Read the model definition and answer for the solid it produces. Units are mm, in the model's axes. A direction names the side the tool comes from. Round coordinates to 2 decimals unless told otherwise and drop trailing zeros. Write each loop counter-clockwise with the first axis right and the second up, starting at its lowest first coordinate (ties: lowest second). Pieces come first, ordered by that corner, then holes. Notation, with made-up numbers: (-3, -18) - (8, -18) arc R5 cw to (8, -10) - close; hole circle Ø5 at (62.5, 84). An arc over 180 degrees is marked (long way). One line per item, written item: value. Start each with the question number.
(1) A cutting plane is placed at B-B, the plane y = 45.5. Determine the outline of the cut face in (x, z), plus the area to 3 significant figures.
(2) A cutting plane is placed at C-C, the plane z = 225. Determine the outline of the cut face in (x, y).
(3) For faces 4 (the face through (9, -170, 0)), 5 (the face through (9, 21.362, -9)), 6 (the face through (9.4, 40.62, 204.85)), 7 (the face through (9, 135, 0)), determine the directions among +Z, -Z, +X, -X, +Y, -Y from which every point of the face is accessible in a straight line to the end or side of a thin tool.
(4) The mould has two halves that part along Y. Classify faces 1 (the face through (9.4, -132.12, 86.95)), 2 (the face through (18.542, 19, 122)), 3 (the face through (9, 97.562, -9)): +Y half, -Y half, draft (parallel to the pull), parting line (faces both ways), or undercut.
(5) Find the intervals of material crossed by L1, parallel to Y at x = 9.75, z = -1; L2, parallel to Y at x = 12.5, z = 92.5; L3, parallel to Z at x = 5, y = -84.5, in increasing order.
(6) A cutting plane is placed at A-A, the plane x = 3.75. Determine the outline of the cut face in (y, z).
(7) Flat-ended cylindrical pins translate along their axes: pin 1 Ø10 at (x, z) = (5, 182) entering from -Y; pin 2 Ø5.5 at (x, y) = (5.5, -161) entering from -Z; pin 3 Ø9.5 at (x, z) = (13, -9) entering from +Y. Find the tip coordinate at first contact, or state that the pin passes through.
(8) A cutting plane is placed at D-D, the plane z = 308. Determine the outline of the cut face in (x, y).
from build123d import *

# Parameters (mm, degrees)
F1_DEPTH = 18.542
F2_W     = 18.542
F2_H     = 76.2
F3_DEPTH = 18.542
F5_DEPTH = 25.4


with BuildPart() as f1:
    # F0 (on Right) → F1 (new body)
    with BuildSketch(Plane.YZ):
        with BuildLine():
            ThreePointArc((-199.645225, 104.186206), (-217.85746, 53.143737), (-207.238496, 0))
            Line((-207.238496, 0), (173.761504, 0))
            Line((173.761504, 0), (173.761504, 330.2))
            ThreePointArc((173.761504, 330.2), (124.464127, 333.733445), (79.332339, 313.588016))
            Line((79.332339, 313.588016), (-199.645225, 104.186206))
        make_face()
    extrude(amount=F1_DEPTH)

    # F2 (on face) → F3 (join)
    with BuildSketch(Plane(origin=(0, 0, 0), x_dir=(1, 0, 0), z_dir=(0, 0, -1))):
        with Locations((9.271, -59.461504)):
            Rectangle(F2_W, F2_H)
        with Locations((9.271, 92.938496)):
            Rectangle(F2_W, F2_H)
    extrude(amount=F3_DEPTH)

    # F4 (on face) → F5 (cut)
    with BuildSketch(Plane.YZ.offset(18.542)):
        Polygon((-5.565468, 193.369503), (5.565468, 178.540207), (76.664833, 231.907709), (65.533897, 246.737005), align=None)
        Polygon((-66.507781, 147.62593), (-137.607146, 94.258428), (-126.47621, 79.429131), (-55.376845, 132.796634), align=None)
    extrude(amount=-F5_DEPTH, mode=Mode.SUBTRACT)


solid = f1.part
Here are the results:
1. outline: (0, -18.54) - (18.54, -18.54) - (18.54, 208.52) - (0, 208.52) - close; (0, 231.7) - (18.54, 231.7) - (18.54, 288.19) - (0, 288.19) - close
1. area: 5,260 mm²
2. outline: (0, -38.69) - (18.54, -38.69) - (18.54, 36.57) - (0, 36.57) - close; (0, 67.46) - (18.54, 67.46) - (18.54, 173.76) - (0, 173.76) - close
3. face 4: -Z, +X, -X, -Y
3. face 5: -Z, +X, -X
3. face 6: +X, -X
3. face 7: -Z, +X, -X, +Y
4. face 1: undercut
4. face 2: draft
4. face 3: +Y half
5. L1: -131.04 to -54.84, 21.36 to 97.56
5. L2: -206.74 to -136.29, -109.06 to 173.76
5. L3: -18.54 to 110.94, 134.12 to 190.61
6. outline: (-207.24, 0) - (-131.04, 0) - (-131.04, -18.54) - (-54.84, -18.54) - (-54.84, 0) - (21.36, 0) - (21.36, -18.54) - (97.56, -18.54) - (97.56, 0) - (173.76, 0) - (173.76, 330.2) arc R101.6 ccw to (79.33, 313.59) - (-199.65, 104.19) arc R101.6 ccw to start; hole (-137.61, 94.26) - (-126.48, 79.43) - (-55.38, 132.8) - (-66.51, 147.63) - close; hole (-5.57, 193.37) - (5.57, 178.54) - (76.66, 231.91) - (65.53, 246.74) - close
7. pin 1: y = -102.64
7. pin 2: z = 0
7. pin 3: y = 97.56
8. outline: (0, 71.89) - (18.54, 71.89) - (18.54, 173.76) - (0, 173.76) - close
